Model file for the job. Use its own axes, mm. A direction names the side the tool comes from. Coordinates: 2 decimals unless noted, no trailing zeros. Loops run counter-clockwise (first coordinate to the right, second up) from the corner with the lowest first, then second, coordinate; pieces in that order, holes last.
from build123d import *

# Parameters (mm, degrees)
SKETCH1_R               = 27
SKETCH1_R_2             = 1.25
SKETCH1_R_3             = 20
BOSS_EXTRUDE1_DEPTH     = 10
SKETCH3_R               = 20
SKETCH3_R_2             = 1.25
BOSS_EXTRUDE2_DEPTH     = 2
SKETCH5_W               = 15
SKETCH5_H               = 24.16646527
BOSS_EXTRUDE3_DEPTH     = 3.5
CUT_EXTRUDE1_REACH      = 59.191
CUT_EXTRUDE1_END_RADIUS = 27
SKETCH4_W               = 6
SKETCH4_H               = 4


with BuildPart() as part:
    # Sketch1 → Boss-Extrude1 (new body)
    with BuildSketch(Plane.XY):
        Circle(SKETCH1_R)
        with Locations((0, 23.5)):
            Circle(SKETCH1_R_2, mode=Mode.SUBTRACT)
        with Locations((23.5, 0)):
            Circle(SKETCH1_R_2, mode=Mode.SUBTRACT)
        with Locations((0, -23.5)):
            Circle(SKETCH1_R_2, mode=Mode.SUBTRACT)
        with Locations((-23.5, 0)):
            Circle(SKETCH1_R_2, mode=Mode.SUBTRACT)
        Circle(SKETCH1_R_3, mode=Mode.SUBTRACT)
    extrude(amount=BOSS_EXTRUDE1_DEPTH)

    # Sketch3 → Boss-Extrude2 (add)
    with BuildSketch(Plane.XY):
        Circle(SKETCH3_R)
        with Locations((-7, 0)):
            Circle(SKETCH3_R_2, mode=Mode.SUBTRACT)
        with Locations((7, 0)):
            Circle(SKETCH3_R_2, mode=Mode.SUBTRACT)
    extrude(amount=BOSS_EXTRUDE2_DEPTH)

    # Sketch5 → Boss-Extrude3 (add)
    with BuildSketch(Plane.XY):
        with Locations((0, 37.331237278)):
            Rectangle(SKETCH5_W, SKETCH5_H)
    extrude(amount=BOSS_EXTRUDE3_DEPTH)

    # Cut-Extrude1: up to this cylinder (the profile starts inside it)
    cut_extrude1_end = Plane(origin=(0, 0, 5.5), z_dir=(0, 0, -1)) * Cylinder(CUT_EXTRUDE1_END_RADIUS, 173.382, mode=Mode.PRIVATE)
    # Sketch4 → Cut-Extrude1 (cut, up to the surface)
    with BuildSketch(Plane(origin=(0, 0, 0), x_dir=(1, 0, 0), z_dir=(0, 1, 0)), mode=Mode.PRIVATE) as cut_extrude1_sk1:
        with Locations((-11, -5.5)):
            Rectangle(SKETCH4_W, SKETCH4_H)
    cut_extrude1_tool1 = extrude(cut_extrude1_sk1.sketch, amount=-CUT_EXTRUDE1_REACH, mode=Mode.PRIVATE) & cut_extrude1_end
    add(cut_extrude1_tool1.solids().sort_by_distance((-11, 0, 5.5))[0], mode=Mode.SUBTRACT)


solid = part.part
Q1. Slice it at B-B (z = 6.5). List the corners of the cut face in (x, y).
Answers:
outline: (-14, -23.09) - (-14, -14.28) arc R20 cw (long way) to (-8, -18.33) - (-8, -25.79) arc R27 ccw (long way) to start; hole circle Ø2.5 at (-23.5, 0); hole circle Ø2.5 at (0, -23.5); hole circle Ø2.5 at (0, 23.5); hole circle Ø2.5 at (23.5, 0)
Q2. Flat gauge pins, fed straight in: P1, Ø3, axis at x = -10, y = -18.5, coming from the -Z side; P2, Ø5, axis at x = -15, z = 4, coming from the -Y side; P3, Ø1.8, axis at y = 38.5, z = 1.5, coming from the +X side; P4, Ø5, axis at x = 20, z = 8, coming from the -Y side. Where does each tip first touch, or does it go through?
Answers:
P1: stops at z = 0
P2: stops at y = -23.91
P3: stops at x = 7.5
P4: stops at y = -20.56
Q3. Mould opens along Z. For faces 5 (the flat face through (-4, -20, 10)), 6 (the flat face through (7.5, 38, 2)), 7 (the flat face through (-11, -20, 7.5)) say: +Z half, -Z half, draft (parallel to the pull), parting line (faces both ways), or undercut.
Answers:
face 5: +Z half
face 6: draft
face 7: undercut
Q4. Slice it at A-A (x = 0). List the corners of the cut face in (y, z).
Answers:
outline: (-27, 0) - (-24.75, 0) - (-24.75, 10) - (-27, 10) - close; (-22.25, 0) - (22.25, 0) - (22.25, 10) - (20, 10) - (20, 2) - (-20, 2) - (-20, 10) - (-22.25, 10) - close; (24.75, 0) - (49.41, 0) - (49.41, 3.5) - (27, 3.5) - (27, 10) - (24.75, 10) - close
Q5. Which spindle directions (+Z, -Z, +X, -X, +Y, -Y) get a long thin tool onto all of the face, cutting with end or side? Do faces 1 (the cylindrical face through (-4.336, -19.524, 5.944)), 2 (the flat face through (-7.5, 38, 2)), 3 (the flat face through (-8, -22, 6)), 4 (the cylindrical face through (-22.345, -0.479, 4.93)). Say none if no direction does.
Answers:
face 1: +Z
face 2: +Z, -Z, -X, +Y
face 3: -Y
face 4: +Z, -Z
Q6. Slice it at C-C (y = 23.5). List the corners of the cut face in (x, z), and give its area (3 significant figures).
Answers:
outline: (-13.29, 0) - (-1.25, 0) - (-1.25, 10) - (-13.29, 10) - close; (1.25, 0) - (13.29, 0) - (13.29, 10) - (1.25, 10) - close
area: 241 mm2
Q7. Drill centre lines: line 1 (Y direction, x = 0, z = 5.25); line 2 (Z direction, x = -14, y = 6.5); line 3 (X direction, y = 1, z = 1). Where is each one in solid material? Low to high.
Answers:
line 1: y = -27 to -24.75, -22.25 to -20, 20 to 22.25, 24.75 to 27
line 2: z = 0 to 2
line 3: x = -26.98 to -24.25, -22.75 to -7.75, -6.25 to 6.25, 7.75 to 22.75, 24.25 to 26.98
Q8. Slice it at D-D (x = -12.5). List the corners of the cut face in (y, z).
Answers:
outline: (-23.93, 0) - (23.93, 0) - (23.93, 10) - (15.61, 10) - (15.61, 2) - (-15.61, 2) - (-15.61, 3.5) - (-23.93, 3.5) - close; (-23.93, 7.5) - (-15.61, 7.5) - (-15.61, 10) - (-23.93, 10) - close
